Input: part model. Units: mm. Frame: model coordinates. A direction names the side the tool comes from. Coordinates: 2 decimals unless noted, no trailing zeros. Write each loop counter-clockwise with the first axis right and the second up, starting at its lowest first coordinate (ties: lowest second). Pieces come first, ordered by that corner, then holes. Notation, with made-up numbers: (46.25, -1) -> (85.25, -1) arc R33 cw to (85.25, 36) -> close; hole circle Ø1 at (70, 22.25). An arc over 180 degrees is marked (long way). Use one line per item in the form item = value. Start each with the question number.
(1) Set-up query: faces 1 (the face through (-8.348, -33, 1)), 2 (the face through (-12.087, 33.3, 10.2)), 3 (the face through (-9.812, -48.657, -10.805)). Return all of +Z, -Z, +X, -X, +Y, -Y with unobstructed straight access to the full face (end or side cutting, diameter ignored); none if empty.
(2) Cut plane D-D on x = -19.5. Return the cut outline in (y, z), plus the area to 3 significant figures.
(3) Cut plane A-A on y = 0. Return the cut outline in (x, z), plus the area to 3 significant figures.
(4) Ray query, line 1 along Z through (x, y) = (15, 1); line 2 along Y through (x, z) = (-32.5, 4); line 3 along Y through (x, z) = (23.5, -5). Return the intervals inside material, ascending.
(5) Cut plane C-C on x = 12.5. Return the cut outline in (y, z).
(6) First-contact query: pin 1 (4 mm diameter, centred on x = 15.5, z = 13, fed in from -Y); pin 2 (6 mm diameter, centred on x = -16.5, z = -13.5, fed in from +Y); pin 3 (2 mm diameter, centred on x = -21.5, y = 17.5, fed in from -Z). Flat tips, straight axial feed; report the tip coordinate or a pass-through.
```python
from build123d import *


with BuildPart() as f1:
    # F0 (on Front) → F1 (revolve)
    with BuildSketch(Plane.XZ):
        with BuildLine():
            Line((-42.988531, 26.665349), (-42.988531, 0))
            Line((-42.988531, 0), (27.039163, 0))
            Line((27.039163, 0), (27.039163, 25.46965))
            ThreePointArc((27.039163, 25.46965), (25.30211, 29.663266), (21.108494, 31.400319))
            Line((21.108494, 31.400319), (-8.348497, 31.400319))
            Line((-8.348497, 31.400319), (-8.348497, 49.841773))
            Line((-8.348497, 49.841773), (-11.235781, 49.841773))
            ThreePointArc((-11.235781, 49.841773), (-11.837422, 49.592565), (-12.08663, 48.990924))
            Line((-12.08663, 48.990924), (-12.08663, 34.614854))
            ThreePointArc((-12.08663, 34.614854), (-12.955154, 32.518051), (-15.051958, 31.649526))
            Line((-15.051958, 31.649526), (-38.004354, 31.649526))
            ThreePointArc((-38.004354, 31.649526), (-41.528699, 30.189694), (-42.988531, 26.665349))
        make_face()
    revolve(axis=Axis((-7.974684, 0, 0), (-1, 0, 0)))


solid = f1.part
```
Values:
q1.face_1 = +X
q1.face_2 = -X
q1.face_3 = +X, -X
q2.outline = circle Ø63.3 at (0, 0)
q2.area = 3,150 mm2
q3.outline = (-42.99, -26.67) arc R4.98 ccw to (-38, -31.65) -> (-15.05, -31.65) arc R2.97 cw to (-12.09, -34.61) -> (-12.09, -48.99) arc R0.85 ccw to (-11.24, -49.84) -> (-8.35, -49.84) -> (-8.35, -31.4) -> (21.11, -31.4) arc R5.93 ccw to (27.04, -25.47) -> (27.04, 25.47) arc R5.93 ccw to (21.11, 31.4) -> (-8.35, 31.4) -> (-8.35, 49.84) -> (-11.24, 49.84) arc R0.85 ccw to (-12.09, 48.99) -> (-12.09, 34.61) arc R2.97 cw to (-15.05, 31.65) -> (-38, 31.65) arc R4.98 ccw to (-42.99, 26.67) -> close
q3.area = 4,530 mm2
q4.line_1 = -31.38 to 31.38
q4.line_2 = -31.4 to 31.4
q4.line_3 = -30.49 to 30.49
q5.outline = circle Ø62.8 at (0, 0)
q6.pin_1 = -29.41
q6.pin_2 = 29.86
q6.pin_3 = -27.01
